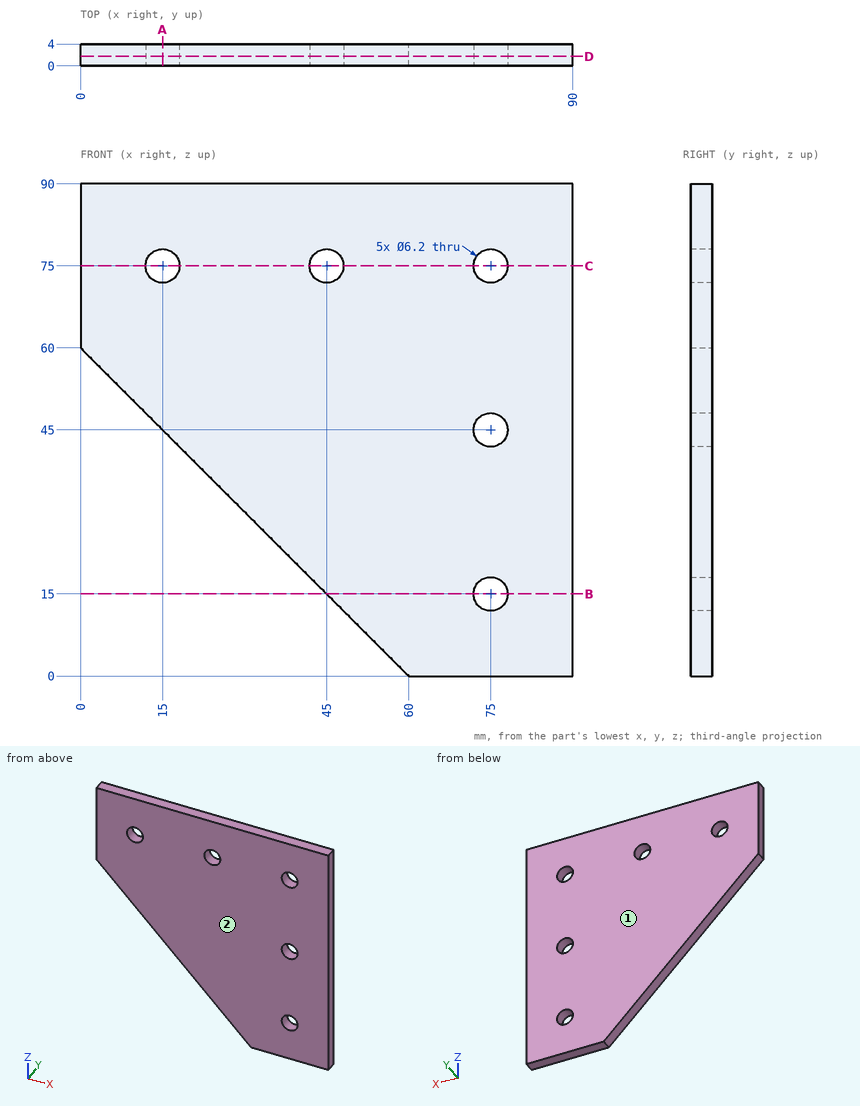
Geometry: see drawing. Coordinates: mm, zero at the bounding-box minimum. Give positions to 0.01 mm unless a question says otherwise; leave off trailing zeros. Loops run counter-clockwise (first coordinate to the right, second up) from the corner with the lowest first, then second, coordinate; pieces in that order, holes last. Notation, with made-up numbers: (48, 17.25) -> (93, 17.25) arc R29 ccw to (93, 48.25) -> close; hole circle Ø3 at (-0.75, 87). An arc over 180 degrees is marked (long way). Answer as a JSON object with one key per item and string values. Group by question number.
Item 1: Cut plane D-D, the plane y = 1.75. Return the cut outline in (x, z), and give its area (3 significant figures).
Item 2: Cut plane C-C, the plane z = 75. Return the cut outline in (x, y), and give its area (3 significant figures).
Item 3: Cut plane B-B, the plane z = 15. Return the cut outline in (x, y).
Item 4: Pin query (flat end, axial travel): P1, Ø3.5, axis at x = 45, z = 75, coming from the +Y side (3 decimals); P2, Ø1.5, axis at x = 18.5, y = 1, coming from the -Z side; P3, Ø1.5, axis at x = 54.5, y = 1.5, coming from the -Z side; P4, Ø1.5, axis at x = 31.5, y = 3, coming from the -Z side. Return the tip coordinate at first contact, or that it passes through.
Item 5: Line query: probe 1 along X at (y, z) = (1.7, 75); probe 2 along Z at (x, y) = (13, 1.35); probe 3 along Z at (x, y) = (44.5, 2.8). Output: solid intervals per line, ascending.
Item 6: Pull-direction query (Y, two-part tool) for the marked faces 1 and 2; classes: released by +Y, released by -Y, zero draft, split by the parting line, or undercut.
Item 7: Cut plane A-A, the plane x = 15. Return the cut outline in (y, z).
Checks:
{
 "1": {"outline": "(0, 60) -> (60, 0) -> (90, 0) -> (90, 90) -> (0, 90) -> close; hole circle Ø6.2 at (15, 75); hole circle Ø6.2 at (45, 75); hole circle Ø6.2 at (75, 15); hole circle Ø6.2 at (75, 45); hole circle Ø6.2 at (75, 75)", "area": "6,150 mm²"},
 "2": {"outline": "(0, 0) -> (11.9, 0) -> (11.9, 4) -> (0, 4) -> close; (18.1, 0) -> (41.9, 0) -> (41.9, 4) -> (18.1, 4) -> close; (48.1, 0) -> (71.9, 0) -> (71.9, 4) -> (48.1, 4) -> close; (78.1, 0) -> (90, 0) -> (90, 4) -> (78.1, 4) -> close", "area": "286 mm²"},
 "3": {"outline": "(45, 0) -> (71.9, 0) -> (71.9, 4) -> (45, 4) -> close; (78.1, 0) -> (90, 0) -> (90, 4) -> (78.1, 4) -> close"},
 "4": {"P1": "passes through", "P2": "stops at z = 40.75", "P3": "stops at z = 4.75", "P4": "stops at z = 27.75"},
 "5": {"probe 1": "x = 0 to 11.9, 18.1 to 41.9, 48.1 to 71.9, 78.1 to 90", "probe 2": "z = 47 to 72.63, 77.37 to 90", "probe 3": "z = 15.5 to 71.94, 78.06 to 90"},
 "6": {"face 1": "released by +Y", "face 2": "released by -Y"},
 "7": {"outline": "(0, 45) -> (4, 45) -> (4, 71.9) -> (0, 71.9) -> close; (0, 78.1) -> (4, 78.1) -> (4, 90) -> (0, 90) -> close"}
}
